from build123d import *

# Parameters (mm, degrees)
TAP_DRILL_FOR_M3_TAP1_D = 2.5


with BuildPart() as part:
    # Sketch1 → Revolve1 (revolve)
    with BuildSketch(Plane.XY, mode=Mode.PRIVATE) as revolve1_sk:
        Polygon((11, 0), (11, 4), (5, 4), (5, 9), (4, 9), (4, -2), (5, -2), (5, 0), align=None)
    revolve(revolve1_sk.sketch.rotate(Axis((0, 0, 0), (0, 1, 0)), 90), axis=Axis((0, 0, 0), (0, 1, 0)))

    # Tap Drill for M3 Tap1 (through all)
    with Locations(Plane(origin=(0, 4, 0), x_dir=(1, 0, 0), z_dir=(0, 1, 0))):
        with Locations((0, 8.25), (8.25, 0), (0, -8.25), (-8.25, 0)):
            Hole(TAP_DRILL_FOR_M3_TAP1_D / 2)


solid = part.part
Can you work these out from the model? Positions are in its coordinate system, mm. A direction names the side the tool comes from. Round coordinates to 2 decimals unless told otherwise and drop trailing zeros. Loops run counter-clockwise (first coordinate to the right, second up) from the corner with the lowest first, then second, coordinate; pieces in that order, holes last. Notation, with made-up numbers: (-8.75, -24) - (27.25, -24) arc R14 cw to (27.25, -15) - close; hole circle Ø11 at (-7, -37.5). An arc over 180 degrees is marked (long way). Use CSV: the item, a comma, the result in double quotes. Start each with the question number.
1) If we section it at B-B on z = 0: Write out the boundary of the cut face in (x, y), plus the area to 3 significant figures.
2) If we section it at C-C on y = 3: Write out the boundary of the cut face in (x, z).
3) If we section it at A-A on x = 0: Write out the boundary of the cut face in (y, z).
4) We'd pull the mould along X, two halves only. Please class faces 4 (the flat face through (5, 4, -2)), 5 (the cylindrical face through (-7, 2, 0)), 6 (the cylindrical face through (0, -1, 5)): released by +X, released by -X, zero draft, split by the parting line, or undercut.
5) For pin 1 Ø10 at (x, z) = (0.5, -1) entering from +Y; pin 2 Ø1.5 at (x, z) = (-7, -0.5) entering from +Y; pin 3 Ø8 at (x, z) = (-8.5, 6.5) entering from -Y; pin 4 Ø4 at (y, z) = (7.5, 3.5) entering from +X, each with a flat end and sliding along its axis, tell me the tip position at first contact or that it passes through.
6) Please list where these lines run through material, in increasing order: probe 1 along X at (y, z) = (1.25, 0.75); probe 2 along Y at (x, z) = (-8.5, -3.5); probe 3 along X at (y, z) = (2.15, 8.25). Write a range as [from, to].
7) For faces 1 (the flat face through (2, 0, 5)), 2 (the cylindrical face through (0.27, 1.97, 9.47)), 3 (the cylindrical face through (0, 7, 5)), which set-ups out of +Z, -Z, +X, -X, +Y, -Y let a thin tool reach every point of the face, with its end or its side?
8) If we section it at D-D on z = -8.25: Write out the boundary of the cut face in (x, y), plus the area to 3 significant figures.
Geometry results:
1,outline,"(-11, 0) - (-9.5, 0) - (-9.5, 4) - (-11, 4) - close; (-7, 0) - (-5, 0) - (-5, -2) - (-4, -2) - (-4, 9) - (-5, 9) - (-5, 4) - (-7, 4) - close; (4, -2) - (5, -2) - (5, 0) - (7, 0) - (7, 4) - (5, 4) - (5, 9) - (4, 9) - close; (9.5, 0) - (11, 0) - (11, 4) - (9.5, 4) - close"
1,area,"50.0 mm2"
2,outline,"circle Ø22 at (0, 0); hole circle Ø2.5 at (-8.25, 0); hole circle Ø8 at (0, 0); hole circle Ø2.5 at (0, -8.25); hole circle Ø2.5 at (0, 8.25); hole circle Ø2.5 at (8.25, 0)"
3,outline,"(-2, -5) - (0, -5) - (0, -7) - (4, -7) - (4, -5) - (9, -5) - (9, -4) - (-2, -4) - close; (-2, 4) - (9, 4) - (9, 5) - (4, 5) - (4, 7) - (0, 7) - (0, 5) - (-2, 5) - close; (0, -11) - (4, -11) - (4, -9.5) - (0, -9.5) - close; (0, 9.5) - (4, 9.5) - (4, 11) - (0, 11) - close"
4,face 4,"zero draft"
4,face 5,"undercut"
4,face 6,"split by the parting line"
5,pin 1,"stops at y = 9"
5,pin 2,"stops at y = 4"
5,pin 3,"stops at y = 0"
5,pin 4,"stops at x = 4.77"
6,probe 1,"x = [-10.97, -9.25], [-7.25, -3.93], [3.93, 7.25], [9.25, 10.97]"
6,probe 2,"y = [0, 4]"
6,probe 3,"x = [-7.28, -1.25], [1.25, 7.28]"
7,face 1,"-Y"
7,face 2,"+Y, -Y"
7,face 3,"+Y"
8,outline,"(-7.28, 0) - (-1.25, 0) - (-1.25, 4) - (-7.28, 4) - close; (1.25, 0) - (7.28, 0) - (7.28, 4) - (1.25, 4) - close"
8,area,"48.2 mm2"
